from build123d import *

# Parameters (mm, degrees)
SKETCH1_W           = 55
SKETCH1_H           = 45
SKETCH1_R           = 2.5
SKETCH1_R_2         = 1.5
BOSS_EXTRUDE1_DEPTH = 4.7625


with BuildPart() as part:
    # Sketch1 → Boss-Extrude1 (new body)
    with BuildSketch(Plane.XY):
        with Locations((27.5, 22.5)):
            Rectangle(SKETCH1_W, SKETCH1_H)
        with Locations(Location((10, 10, 0), (0, 0, 180))):
            Circle(SKETCH1_R, mode=Mode.SUBTRACT)
        with Locations(Location((30.5, 30, 0), (0, 0, 180))):
            Circle(SKETCH1_R_2, mode=Mode.SUBTRACT)
        with Locations(Location((49.5, 30, 0), (0, 0, 180))):
            Circle(SKETCH1_R_2, mode=Mode.SUBTRACT)
        with Locations(Location((40, 38, 0), (0, 0, 180))):
            Circle(SKETCH1_R_2, mode=Mode.SUBTRACT)
        with Locations(Location((40, 22, 0), (0, 0, 180))):
            Circle(SKETCH1_R_2, mode=Mode.SUBTRACT)
    extrude(amount=BOSS_EXTRUDE1_DEPTH)


solid = part.part
For this review, take the finished solid that the model builds, in its own axes (mm). Round coordinates to 2 decimals unless told otherwise and drop trailing zeros. Order: outer loops, then holes, each group sorted by start corner. A loop starts at its lowest first (then second) coordinate and runs counter-clockwise, first axis right, second up. Notation, with made-up numbers: (-30.75, 29.25) -> (6.25, 29.25) arc R24 cw to (6.25, 46.25) -> close; hole circle Ø6 at (-6, 1.25). An arc over 180 degrees is marked (long way). Put each result on its own line as item: value.
Q1. Add section B-B on x = 30.5. Write out the cut boundary in (y, z), plus the area to 3 significant figures.
Check result:
outline: (0, 0) -> (28.5, 0) -> (28.5, 4.76) -> (0, 4.76) -> close; (31.5, 0) -> (45, 0) -> (45, 4.76) -> (31.5, 4.76) -> close
area: 200 mm2
Q2. Add section C-C on x = 40. Write out the cut boundary in (y, z).
Check result:
outline: (0, 0) -> (20.5, 0) -> (20.5, 4.76) -> (0, 4.76) -> close; (23.5, 0) -> (36.5, 0) -> (36.5, 4.76) -> (23.5, 4.76) -> close; (39.5, 0) -> (45, 0) -> (45, 4.76) -> (39.5, 4.76) -> close
Q3. For probe 1 along X at (y, z) = (30, 2.65); probe 2 along Y at (x, z) = (40, 2.55); probe 3 along Y at (x, z) = (30.5, 3.2), list the stretches that pass through material, from the lowest coordinate up. Write a range as [from, to].
Check result:
probe 1: [0, 29], [32, 48], [51, 55]
probe 2: [0, 20.5], [23.5, 36.5], [39.5, 45]
probe 3: [0, 28.5], [31.5, 45]
Q4. Add section A-A on y = 30. Write out the cut boundary in (x, z), plus the area to 3 significant figures.
Check result:
outline: (0, 0) -> (29, 0) -> (29, 4.76) -> (0, 4.76) -> close; (32, 0) -> (48, 0) -> (48, 4.76) -> (32, 4.76) -> close; (51, 0) -> (55, 0) -> (55, 4.76) -> (51, 4.76) -> close
area: 233 mm2
Q5. Add section D-D on y = 10. Write out the cut boundary in (x, z).
Check result:
outline: (0, 0) -> (7.5, 0) -> (7.5, 4.76) -> (0, 4.76) -> close; (12.5, 0) -> (55, 0) -> (55, 4.76) -> (12.5, 4.76) -> close
Q6. Mouldability with a two-part tool opening along Y and no side actions: class faces 1 (the flat face through (27, 45, 2)), 2 (the flat face through (0, 22, 2)), 3 (the cylindrical face through (41.11, 20.99, 2.35)), 4 (the cylindrical face through (50.61, 28.99, 2.35)) as pulls with the +Y half, pulls with the -Y half, needs draft (parallel to the pull), parting line crosses it, or undercut.
Check result:
face 1: pulls with the +Y half
face 2: needs draft
face 3: undercut
face 4: undercut
Q7. Insertion check: pin 1 Ø8 at (x, y) = (10, 10) entering from -Z; pin 2 Ø2.5 at (x, y) = (30.5, 30) entering from +Z. Each pin has a flat end and moves straight along its axis. Give the tip position at first contact, or say it passes through.
Check result:
pin 1: z = 0
pin 2: through
